Could you check a few things on this model? Use its own coordinates, in mm. A direction names the side the tool comes from. Give positions to 0.01 mm unless a question says otherwise; leave off trailing zeros. Order: outer loops, then holes, each group sorted by start corner. A loop starts at its lowest first (then second) coordinate and runs counter-clockwise, first axis right, second up. Notation, with made-up numbers: (-16, 89) - (7, 89) arc R21 ccw to (7, 119) - close; hole circle Ø9 at (21, 25.25). An arc over 180 degrees is marked (long way). Put each result on its own line as item: value.
Autodesk Inventor part; units mm, degrees
ref_plane "YZ Plane" through (0, 0, 0) normal (1, 0, 0) x (0, 1, 0)
ref_plane "XZ Plane" through (0, 0, 0) normal (0, 1, 0) x (-1, 0, 0)
ref_plane "XY Plane" through (0, 0, 0) normal (0, 0, 1) x (1, 0, 0)
sketch "Sketch1" plane through (0, 0, 0) normal (0, 1, 0) x (-1, 0, 0)
  line L0 (-2.9762, 2.1033) -> (4.0238, 2.1033)
  line L1 (4.0238, 2.1033) -> (4.0238, -4.8967)
  line L2 (4.0238, -4.8967) -> (-2.9762, -4.8967)
  line L3 (-2.9762, -4.8967) -> (-2.9762, 2.1033)
  point P0 (0, 0)
  dimension "d0" = 7
  dimension "d1" = 7
extrude "Extrusion1" add sketch "Sketch1" along normal blind 2
sketch "Sketch2" plane through (0, 2, 0) normal (0, 1, 0) x (1, 0, 0)
  circle A0 centre (-0.5238, 1.3967) radius 2.03
  point P0 (0, 0)
  dimension "d4" = 4.06
extrude "Extrusion2" add sketch "Sketch2" along normal blind 7.53
properties part number "SMA_Up"
1) Suppose I cut it at C-C, the plane y = 3.5. List the corners of the cut face in (x, z) for me.
Filled in:
outline: circle Ø4.06 at (-0.52, -1.4)
2) If I drill on line 1 (X direction, y = 9, z = -1.5); line 2 (Y direction, x = -3.5, z = 1.5); line 3 (X direction, y = 6.25, z = -2), over which ranges is the centre line in solid material (lowest first)? Write a range as [from, to].
Filled in:
line 1: x = [-2.55, 1.5]
line 2: y = [0, 2]
line 3: x = [-2.46, 1.41]
3) Suppose I cut it at B-B, the plane z = -3.25. List the corners of the cut face in (x, y) for me, and give its area (3 significant figures).
Filled in:
outline: (-4.02, 0) - (2.98, 0) - (2.98, 2) - (0.3, 2) - (0.3, 9.53) - (-1.35, 9.53) - (-1.35, 2) - (-4.02, 2) - close
area: 26.5 mm^2
4) I'm going to push flat-ended pins straight in: pin 1 (1.5 mm diameter, centred on y = 6.5, z = -1, fed in from -X); pin 2 (1 mm diameter, centred on x = -2, z = -0.5, fed in from -Y); pin 3 (1.5 mm diameter, centred on y = 7.5, z = -2, fed in from +X); pin 4 (4 mm diameter, centred on x = -1, y = 4.5, fed in from +Z). Where does each tip first touch, or does it pass through?
Filled in:
pin 1: stops at x = -2.55
pin 2: stops at y = 0
pin 3: stops at x = 1.51
pin 4: stops at z = 0.63
5) Suppose I cut it at D-D, the plane z = 1. List the corners of the cut face in (x, y) for me, and give its area (3 significant figures).
Filled in:
outline: (-4.02, 0) - (2.98, 0) - (2.98, 2) - (-4.02, 2) - close
area: 14.0 mm^2
6) Suppose I cut it at A-A, the plane x = -0.75. List the corners of the cut face in (y, z) for me.
Filled in:
outline: (0, -4.9) - (2, -4.9) - (2, -3.41) - (9.53, -3.41) - (9.53, 0.62) - (2, 0.62) - (2, 2.1) - (0, 2.1) - close
7) Which directions (+Z, -Z, +X, -X, +Y, -Y) give clear straight access to the entire face, cutting with the end or side of a thin tool? Please do faces 1 (the flat face through (0, 1, 2.103)), 2 (the cylindrical face through (-0.96, 5.71, -3.38)).
Filled in:
face 1: +Z, +X, -X, +Y, -Y
face 2: +Y
